Geometry: final body of the model. Coordinates: model frame, mm. Round coordinates to 2 decimals unless told otherwise and drop trailing zeros. Loops run counter-clockwise (first coordinate to the right, second up) from the corner with the lowest first, then second, coordinate; pieces in that order, holes last. Notation, with made-up numbers: (-37, 13) -> (-32, 13) arc R29 ccw to (-32, 46) -> close; hole circle Ø5 at (74.5, 26.25). An arc over 180 degrees is marked (long way). Answer in a Markdown table with one row per item.
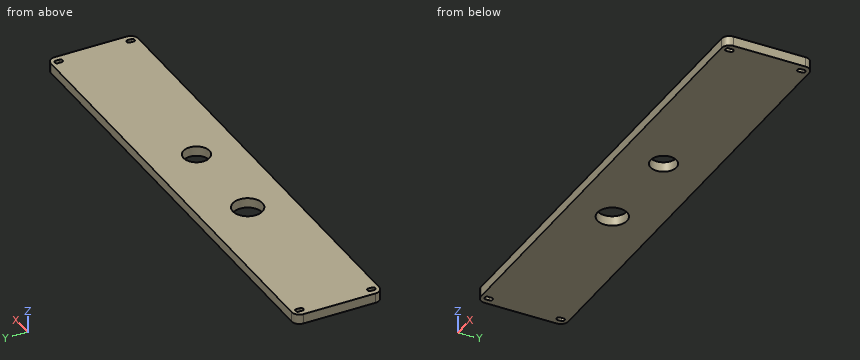
```python
from build123d import *

# Parameters (mm, degrees)
SKETCH1_W           = 607.568
SKETCH1_H           = 112.522
SKETCH1_R           = 16.65
SKETCH1_R_2         = 19
BOSS_EXTRUDE1_DEPTH = 12.7
FILLET1_R           = 10


with BuildPart() as part:
    # Sketch1 → Boss-Extrude1 (new body)
    with BuildSketch(Plane.XY):
        with Locations((40.068414536, 75.801223419)):
            Rectangle(SKETCH1_W, SKETCH1_H)
        with Locations((88.632564672, 74.018682095)):
            Circle(SKETCH1_R, mode=Mode.SUBTRACT)
        with Locations((-36.367435328, 74.018682095)):
            Circle(SKETCH1_R_2, mode=Mode.SUBTRACT)
        with BuildLine():
            Line((334.352414536, 24.540223419), (333.352414536, 24.540223419))
            ThreePointArc((333.352414536, 24.540223419), (331.584647583, 25.272456466), (330.852414536, 27.040223419))
            Line((330.852414536, 27.040223419), (330.852414536, 32.040223419))
            ThreePointArc((330.852414536, 32.040223419), (331.584647583, 33.807990372), (333.352414536, 34.540223419))
            Line((333.352414536, 34.540223419), (334.352414536, 34.540223419))
            ThreePointArc((334.352414536, 34.540223419), (336.120181489, 33.807990372), (336.852414536, 32.040223419))
            Line((336.852414536, 32.040223419), (336.852414536, 27.040223419))
            ThreePointArc((336.852414536, 27.040223419), (336.120181489, 25.272456466), (334.352414536, 24.540223419))
        make_face(mode=Mode.SUBTRACT)
        with BuildLine():
            Line((-253.217585464, 24.540223419), (-254.217585464, 24.540223419))
            ThreePointArc((-254.217585464, 24.540223419), (-255.985352417, 25.272456466), (-256.717585464, 27.040223419))
            Line((-256.717585464, 27.040223419), (-256.717585464, 32.040223419))
            ThreePointArc((-256.717585464, 32.040223419), (-255.985352417, 33.807990372), (-254.217585464, 34.540223419))
            Line((-254.217585464, 34.540223419), (-253.217585464, 34.540223419))
            ThreePointArc((-253.217585464, 34.540223419), (-251.449818511, 33.807990372), (-250.717585464, 32.040223419))
            Line((-250.717585464, 32.040223419), (-250.717585464, 27.040223419))
            ThreePointArc((-250.717585464, 27.040223419), (-251.449818511, 25.272456466), (-253.217585464, 24.540223419))
        make_face(mode=Mode.SUBTRACT)
        with BuildLine():
            Line((-253.217585464, 117.060223419), (-254.217585464, 117.060223419))
            ThreePointArc((-254.217585464, 117.060223419), (-255.985352417, 117.792456466), (-256.717585464, 119.560223419))
            Line((-256.717585464, 119.560223419), (-256.717585464, 124.560223419))
            ThreePointArc((-256.717585464, 124.560223419), (-255.985352417, 126.327990372), (-254.217585464, 127.060223419))
            Line((-254.217585464, 127.060223419), (-253.217585464, 127.060223419))
            ThreePointArc((-253.217585464, 127.060223419), (-251.449818511, 126.327990372), (-250.717585464, 124.560223419))
            Line((-250.717585464, 124.560223419), (-250.717585464, 119.560223419))
            ThreePointArc((-250.717585464, 119.560223419), (-251.449818511, 117.792456466), (-253.217585464, 117.060223419))
        make_face(mode=Mode.SUBTRACT)
        with BuildLine():
            Line((334.352414536, 117.060223419), (333.352414536, 117.060223419))
            ThreePointArc((333.352414536, 117.060223419), (331.584647583, 117.792456466), (330.852414536, 119.560223419))
            Line((330.852414536, 119.560223419), (330.852414536, 124.560223419))
            ThreePointArc((330.852414536, 124.560223419), (331.584647583, 126.327990372), (333.352414536, 127.060223419))
            Line((333.352414536, 127.060223419), (334.352414536, 127.060223419))
            ThreePointArc((334.352414536, 127.060223419), (336.120181489, 126.327990372), (336.852414536, 124.560223419))
            Line((336.852414536, 124.560223419), (336.852414536, 119.560223419))
            ThreePointArc((336.852414536, 119.560223419), (336.120181489, 117.792456466), (334.352414536, 117.060223419))
        make_face(mode=Mode.SUBTRACT)
    extrude(amount=BOSS_EXTRUDE1_DEPTH)

    # Fillet1
    fillet1_edges = [part.edges().sort_by_distance(p)[0] for p in [
        (-263.715585464, 132.062223419, 6.35),
        (-263.715585464, 19.540223419, 6.35),
        (343.852414536, 19.540223419, 6.35),
        (343.852414536, 132.062223419, 6.35),
    ]]
    fillet(fillet1_edges, radius=FILLET1_R)


solid = part.part
```
Item 1: Ray query, L1, parallel to X at y = 121.5, z = 2.5; L2, parallel to X at y = 74.5, z = 9; L3, parallel to Y at x = 88, z = 1. Return the intervals inside material, ascending.
Ans:
| item | result |
|---|---|
| L1 | -263.72 to -256.72, -250.72 to 330.85, 336.85 to 343.85 |
| L2 | -263.72 to -55.36, -17.37 to 71.99, 105.28 to 343.85 |
| L3 | 19.54 to 57.38, 90.66 to 132.06 |
Item 2: Section query B-B, the plane z = 7. State how many separate pieces and enclosed holes the cut face has, and give its area (3 significant figures).
Ans:
| item | result |
|---|---|
| separate pieces | 1 |
| enclosed holes | 6 |
| area | 66,100 mm2 |
Item 3: First-contact query: P1, Ø1.5, axis at y = 29, z = 3.5, coming from the +X side; P2, Ø1.5, axis at y = 123, z = 7.5, coming from the -X side. Flat tips, straight axial feed; report the tip coordinate or a pass-through.
Ans:
| item | result |
|---|---|
| P1 | x = 343.85 |
| P2 | x = -263.71 |
Item 4: Section query A-A, the plane x = 89.5. Output: boundary loops of the cut face in (y, z), and give its area (3 significant figures).
Ans:
| item | result |
|---|---|
| outline | (19.54, 0) -> (57.39, 0) -> (57.39, 12.7) -> (19.54, 12.7) -> close; (90.65, 0) -> (132.06, 0) -> (132.06, 12.7) -> (90.65, 12.7) -> close |
| area | 1,010 mm2 |
